Source: CAD feature listing. Evaluate the final solid. Frame: model axes, mm. Face numbers are marked on the shaded views. A direction names the side the tool comes from. Give positions to 0.01 mm unless a question says otherwise; leave off trailing zeros. Order: outer loops, then holes, each group sorted by start corner. A loop starts at its lowest first (then second) coordinate and runs counter-clockwise, first axis right, second up. Notation, with made-up numbers: (-24.5, 28) - (3.5, 28) arc R14 ccw to (3.5, 48) - close; hole circle Ø6 at (43.25, 4.5). An arc over 180 degrees is marked (long way). Write each question's results on one line, items separated by ' | '. Start each with the question number.
Item 1: Section D-D on x = 21. Output: boundary loops of the cut face in (y, z), and give its area (3 significant figures).
Item 2: Contact query for flat-ended pins moving along their axis: pin 1 Ø1.5 at (x, y) = (21, 19) entering from +Z; pin 2 Ø2 at (y, z) = (36, 11.5) entering from -X; pin 3 Ø7.5 at (x, z) = (100, 8) entering from -Y. Output: stop coordinate, or through.
Item 3: Section B-B on x = 97. Output: boundary loops of the cut face in (y, z).
Item 4: Line query: line 1 along Y through (x, z) = (8, 1.6); line 2 along Y through (x, z) = (97, 3.7); line 3 along Y through (x, z) = (8, 10.75). Output: solid intervals per line, ascending.
Item 5: Section A-A on y = 59.5. Output: boundary loops of the cut face in (x, z).
Item 6: Section C-C on z = 2. Output: boundary loops of the cut face in (x, y).
Item 7: Set-up query: the marked faces 1 and 2. Return all of +Z, -Z, +X, -X, +Y, -Y with unobstructed straight access to the full face (end or side cutting, diameter ignored); none if empty.
Item 8: Mould query, pull axis Y, two halves, no side actions, for the marked faces 3, 4 and 5. Classes: released by +Y, released by -Y, zero draft, split by the parting line, or undercut.
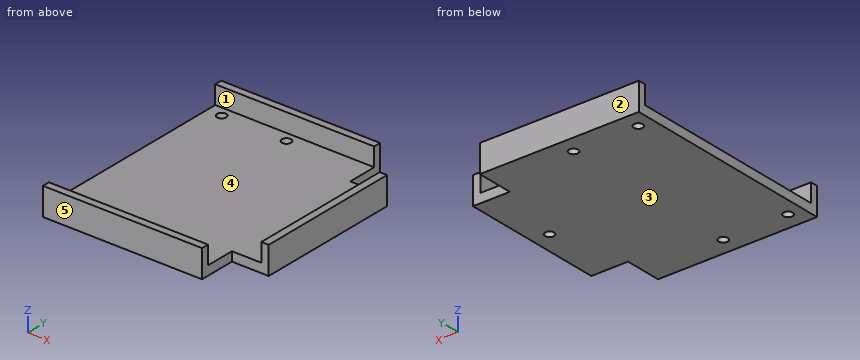
Autodesk Inventor part; units mm, degrees
ref_plane "YZ Plane" through (0, 0, 0) normal (1, 0, 0) x (0, 1, 0)
ref_plane "XZ Plane" through (0, 0, 0) normal (0, 1, 0) x (-1, 0, 0)
ref_plane "XY Plane" through (0, 0, 0) normal (0, 0, 1) x (1, 0, 0)
sketch "Sketch1" plane through (0, 0, 0) normal (0, 0, 1) x (1, 0, 0)
  line L0 (0, 0) -> (106.5, 0) construction
  line L1 (106.5, 0) -> (106.5, 119) construction
  line L2 (106.5, 119) -> (0, 119) construction
  line L3 (0, 119) -> (0, 0) construction
  line L4 (106.5, 119) -> (86.5, 119) construction
  line L5 (86.5, 119) -> (86.5, 99) construction
  line L6 (86.5, 99) -> (106.5, 99) construction
  line L7 (106.5, 99) -> (106.5, 119) construction
  line L8 (106.5, 0) -> (86.5, 0) construction
  line L9 (86.5, 0) -> (86.5, 20) construction
  line L10 (86.5, 20) -> (106.5, 20) construction
  line L11 (106.5, 20) -> (106.5, 0) construction
  line L12 (0, 119) -> (86.5, 119)
  line L13 (86.5, 119) -> (86.5, 99)
  line L14 (86.5, 99) -> (106.5, 99)
  line L15 (106.5, 20) -> (86.5, 20)
  line L16 (86.5, 0) -> (86.5, 20)
  line L17 (86.5, 0) -> (0, 0)
  line L18 (0, 0) -> (0, 119)
  line L19 (106.5, 99) -> (106.5, 20)
  dimension "d0" = 106.5
  dimension "d1" = 119
  dimension "d2" = 20
  dimension "d3" = 20
  dimension "d4" = 20
  dimension "d5" = 20
extrude "Extrusion1" add sketch "Sketch1" along normal blind 5
sketch "Sketch2" plane through (0, 0, 5) normal (0, 0, 1) x (1, 0, 0)
  circle A0 centre (43.25, 9.5) radius 2.5
  circle A1 centre (97, 59.5) radius 2.5
  circle A2 centre (43.25, 109.5) radius 2.5
  line L0 (86.5, 119) -> (0, 119)
  line L1 (0, 0) -> (86.5, 0)
  line L2 (106.5, 20) -> (106.5, 99)
  circle A3 centre (8, 109.5) radius 2.5
  circle A4 centre (8, 9.5) radius 2.5
  line L3 (0, 119) -> (0, 0)
  point P0 (106.5, 59.5)
  point P1 (43.25, 119)
  point P2 (43.25, 0)
  dimension "d8" = 5
  dimension "d9" = 5
  dimension "d10" = 5
  dimension "d11" = 9.5
  dimension "d12" = 9.5
  dimension "d13" = 9.5
  dimension "d21" = 5
  dimension "d22" = 5
  dimension "d23" = 8
extrude "Extrusion2" cut sketch "Sketch2" against normal through all
sketch "Sketch3" plane through (0, 0, 5) normal (0, 0, 1) x (1, 0, 0)
  line L0 (86.5, 119) -> (0, 119)
  line L1 (86.5, 99) -> (86.5, 119)
  line L2 (106.5, 99) -> (86.5, 99)
  line L3 (106.5, 20) -> (106.5, 99)
  line L4 (86.5, 20) -> (106.5, 20)
  line L5 (86.5, 0) -> (86.5, 20)
  line L6 (0, 0) -> (86.5, 0)
  line L7 (0, 115) -> (82.5, 115)
  line L8 (82.5, 115) -> (82.5, 95)
  line L9 (82.5, 95) -> (102.5, 95)
  line L10 (102.5, 95) -> (102.5, 24)
  line L11 (102.5, 24) -> (82.5, 24)
  line L12 (82.5, 24) -> (82.5, 4)
  line L13 (82.5, 4) -> (0, 4)
  line L14 (0, 119) -> (0, 115)
  line L15 (0, 119) -> (0, 0)
  line L16 (0, 4) -> (0, 0)
  dimension "d16" = 4
extrude "Extrusion3" add sketch "Sketch3" along normal blind 10 contours L1 L2 L3 L4 L5 L6 L15 L13 L12 L11 L10 L9 L8 L7 L14 L0
sketch "Sketch4" plane through (0, 0, 15) normal (0, 0, 1) x (1, 0, 0)
  line L0 (82.5, 115) -> (0, 115)
  line L1 (82.5, 115) -> (102.5, 115)
  line L2 (102.5, 115) -> (102.5, 4)
  line L3 (102.5, 4) -> (82.5, 4)
  line L4 (82.5, 4) -> (82.5, 115)
  point P0 (0, 0)
  point P1 (102.5, 95)
extrude "Extrusion4" cut sketch "Sketch4" against normal blind 10
properties part number "BB001" material "ABS Plastic"
Evaluation:
1) outline: (0, 0) - (119, 0) - (119, 15) - (115, 15) - (115, 5) - (4, 5) - (4, 15) - (0, 15) - close | area: 675 mm^2
2) pin 1: stops at z = 5 | pin 2: stops at x = 102.5 | pin 3: stops at y = 20
3) outline: (20, 0) - (57, 0) - (57, 5) - (20, 5) - close; (62, 0) - (99, 0) - (99, 5) - (62, 5) - close
4) line 1: y = 0 to 7, 12 to 107, 112 to 119 | line 2: y = 20 to 57, 62 to 99 | line 3: y = 0 to 4, 115 to 119
5) outline: (0, 0) - (94.5, 0) - (94.5, 5) - (0, 5) - close; (99.5, 0) - (106.5, 0) - (106.5, 15) - (102.5, 15) - (102.5, 5) - (99.5, 5) - close
6) outline: (0, 0) - (86.5, 0) - (86.5, 20) - (106.5, 20) - (106.5, 99) - (86.5, 99) - (86.5, 119) - (0, 119) - close; hole circle Ø5 at (8, 9.5); hole circle Ø5 at (8, 109.5); hole circle Ø5 at (43.25, 9.5); hole circle Ø5 at (43.25, 109.5); hole circle Ø5 at (97, 59.5)
7) face 1: +Z, +X, -X | face 2: +Z, -Z, +X, -X, +Y
8) face 3: zero draft | face 4: undercut | face 5: released by -Y
